```python
from build123d import *

# Parameters (mm, degrees)
F0_W     = 95
F0_H     = 105
F0_R     = 4.25
F1_DEPTH = 8
F2_SIZE  = 0.5


with BuildPart() as f1:
    # F0 (on Front) → F1 (new body)
    with BuildSketch(Plane.XZ):
        with Locations((2.5, 0)):
            Rectangle(F0_W, F0_H)
        with Locations((-27.5, -40)):
            Circle(F0_R, mode=Mode.SUBTRACT)
        with Locations((32.5, -40)):
            Circle(F0_R, mode=Mode.SUBTRACT)
        with Locations((-27.5, 0)):
            Circle(F0_R, mode=Mode.SUBTRACT)
        with Locations((-27.5, 40)):
            Circle(F0_R, mode=Mode.SUBTRACT)
        with Locations((32.5, 0)):
            Circle(F0_R, mode=Mode.SUBTRACT)
        with Locations((32.5, 40)):
            Circle(F0_R, mode=Mode.SUBTRACT)
    extrude(amount=F1_DEPTH)

    # F2
    f2_edges = [f1.edges().sort_by_distance(p)[0] for p in [
        (-31.75, -8, 40),
        (28.25, -8, 40),
        (28.25, -8, -40),
        (-31.75, -8, -40),
        (-31.75, -8, 0),
        (28.25, -8, 0),
    ]]
    chamfer(f2_edges, length=F2_SIZE)


solid = f1.part
```
Work out the finished part from the listing and answer in its coordinate system (mm). Round coordinates to 2 decimals unless told otherwise and drop trailing zeros. Write each loop counter-clockwise with the first axis right and the second up, starting at its lowest first coordinate (ties: lowest second). Pieces come first, ordered by that corner, then holes. Notation, with made-up numbers: (55.5, -4) - (93.5, -4) arc R10 cw to (93.5, 11) - close; hole circle Ø10 at (43.5, 29.25). An arc over 180 degrees is marked (long way). Return JSON: item names as keys, results as strings. Group by question number.
Q1. The part is cut by section C-C on y = -5.5. Write down the section's boundary in (x, z), then the cut area to 3 significant figures.
Q2. The part is cut by section D-D on x = -28. Count the separate pieces of the cut face and the enclosed holes in it, then the cut area to 3 significant figures.
Q3. The part is cut by section B-B on z = -40. Write down the section's boundary in (x, y).
Q4. The part is cut by section A-A on x = 32.5. Write down the section's boundary in (y, z), then the cut area to 3 significant figures.
Q5. This flat-tipped pin is pushed along its axis until it touches: pin 1 Ø10 at (x, z) = (32.5, 40) entering from -Y. Where does it stop, or does it pass through?
Q6. Find the intervals of material crossed by L1, parallel to Z at x = 32.5, y = -4; L2, parallel to Z at x = -25.5, y = -3.25; L3, parallel to X at y = -0.5, z = 43, in increasing order.
Q7. The mould has two halves that part along X. Classify faces 1 (the cylindrical face through (-31.746, -3.698, 0.187)), 2 (the flat face through (-45, -4, -1)), 3 (the flat face through (50, -4, -1)): released by +X, released by -X, zero draft, split by the parting line, or undercut.
Solved:
{
 "1": {"outline": "(-45, -52.5) - (50, -52.5) - (50, 52.5) - (-45, 52.5) - close; hole circle Ø8.5 at (-27.5, -40); hole circle Ø8.5 at (-27.5, 0); hole circle Ø8.5 at (-27.5, 40); hole circle Ø8.5 at (32.5, -40); hole circle Ø8.5 at (32.5, 0); hole circle Ø8.5 at (32.5, 40)", "area": "9,630 mm²"},
 "2": {"separate pieces": "4", "enclosed holes": "0", "area": "637 mm²"},
 "3": {"outline": "(-45, -8) - (-32.25, -8) - (-31.75, -7.5) - (-31.75, 0) - (-45, 0) - close; (-23.25, -7.5) - (-22.75, -8) - (27.75, -8) - (28.25, -7.5) - (28.25, 0) - (-23.25, 0) - close; (36.75, -7.5) - (37.25, -8) - (50, -8) - (50, 0) - (36.75, 0) - close"},
 "4": {"outline": "(-8, -52.5) - (0, -52.5) - (0, -44.25) - (-7.5, -44.25) - (-8, -44.75) - close; (-8, -35.25) - (-7.5, -35.75) - (0, -35.75) - (0, -4.25) - (-7.5, -4.25) - (-8, -4.75) - close; (-8, 4.75) - (-7.5, 4.25) - (0, 4.25) - (0, 35.75) - (-7.5, 35.75) - (-8, 35.25) - close; (-8, 44.75) - (-7.5, 44.25) - (0, 44.25) - (0, 52.5) - (-8, 52.5) - close", "area": "635 mm²"},
 "5": {"pin 1": "y = -8"},
 "6": {"L1": "-52.5 to -44.25, -35.75 to -4.25, 4.25 to 35.75, 44.25 to 52.5", "L2": "-52.5 to -43.75, -36.25 to -3.75, 3.75 to 36.25, 43.75 to 52.5", "L3": "-45 to -30.51, -24.49 to 29.49, 35.51 to 50"},
 "7": {"face 1": "undercut", "face 2": "released by -X", "face 3": "released by +X"}
}
